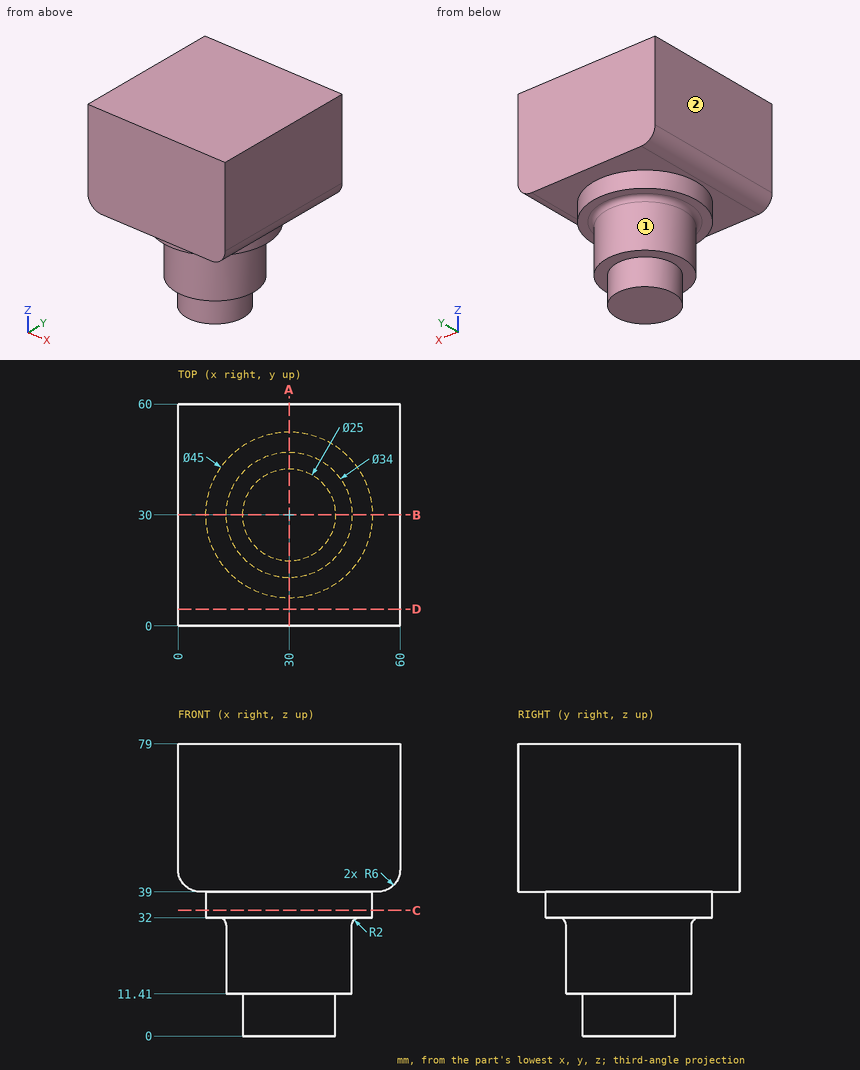
Input: dimensioned drawing with shaded views. Units: mm. Origin: part minimum x, y, z. A direction names the side the tool comes from. Give positions to 0.01 mm unless a question says otherwise; leave off trailing zeros. Write each loop counter-clockwise with the first axis right and the second up, starting at its lowest first coordinate (ties: lowest second). Pieces come first, ordered by that corner, then holes. Notation, with made-up numbers: M 63,18.25 L 119,18.25 A9 cw 119,27.25 Z; hole C 78.25,33.25 d11. An arc over 180 degrees is marked long. Write item = value, one per line. Start each with the question number.
1) Cut plane A-A on x = 30. Return the cut outline in (y, z), then the cut area to 3 significant figures.
2) First-contact query: pin 1 Ø1 at (x, y) = (48.5, 9.5) entering from -Z. Flat tip, straight axial feed; report the tip coordinate or a pass-through.
3) Material intervals for line 1 along Z through (x, y) = (35, 6); line 2 along Y through (x, z) = (29.5, 20.5); line 3 along Z through (x, y) = (31.5, 8.5), sorted ascending. Write a range as [from, to].
4) Cut plane D-D on y = 4.5. Return the cut outline in (x, z).
5) Cut plane C-C on z = 34. Return the cut outline in (x, y).
6) Cut plane B-B on y = 30. Return the cut outline in (x, z).
7) Reachability of the marked faces 1 and 2 from +Z, -Z, +X, -X, +Y, -Y: full face, straight path, thin tool, end or side. Return the list, or none.
Solved:
q1.outline = M 0,39 L 7.5,39 L 7.5,32 L 11,32 A2 cw 13,30 L 13,11.41 L 17.5,11.41 L 17.5,0 L 42.5,0 L 42.5,11.41 L 47,11.41 L 47,30 A2 cw 49,32 L 52.5,32 L 52.5,39 L 60,39 L 60,79 L 0,79 Z
q1.area = 3,700 mm2
q2.pin_1 = 39
q3.line_1 = [39, 79]
q3.line_2 = [13.01, 46.99]
q3.line_3 = [32, 79]
q4.outline = M 0,45 A6 ccw 6,39 L 54,39 A6 ccw 60,45 L 60,79 L 0,79 Z
q5.outline = C 30,30 d45
q6.outline = M 0,45 A6 ccw 6,39 L 7.5,39 L 7.5,32 L 11,32 A2 cw 13,30 L 13,11.41 L 17.5,11.41 L 17.5,0 L 42.5,0 L 42.5,11.41 L 47,11.41 L 47,30 A2 cw 49,32 L 52.5,32 L 52.5,39 L 54,39 A6 ccw 60,45 L 60,79 L 0,79 Z
q7.face_1 = -Z
q7.face_2 = +Z, -Z, -X, +Y, -Y
